Autodesk Inventor part; units mm, degrees
ref_plane "Work Plane1" through (0, 0, 0) normal (0, 0.5, 0.866) x (1, 0, 0)
ref_plane "YZ Plane" through (0, 0, 0) normal (1, 0, 0) x (0, 1, 0)
ref_plane "XZ Plane" through (0, 0, 0) normal (0, 1, 0) x (-1, 0, 0)
sketch "Sketch1" plane through (0, 0, 0) normal (0, 0, 1) x (1, 0, 0)
  line L0 (-1.7498, 0) -> (30, 0)
  line L1 (30, 0) -> (30, 7)
  line L2 (30, 7) -> (2, 7)
  line L3 (2, 7) -> (0.7731, 6.4585)
  line L4 (0.7731, 6.4585) -> (0.45, 6.4585)
  line L5 (0, 6.9085) -> (0, 10.5)
  line L6 (0, 10.5) -> (-9, 10.5)
  line L7 (-9, 10.5) -> (-9, 5.6295)
  line L8 (-9, 5.6295) -> (-5, 5.6295)
  line L9 (-5, 5.6295) -> (-1.7498, 0)
  line L10 (-16.8, 0) -> (37.8, 0)
  line L11 (0, -2.1) -> (0, 12.6)
  line L12 (2, 7) -> (0, 7) construction
  arc A0 (0, 6.9085) -> (0.45, 6.4585) centre (0.45, 6.9085) ccw
  line L13 (0, 10.5) -> (-9, 9.7126)
  point P0 (0, 6.4585)
  dimension "d1" = 28
  dimension "d2" = 1.2269
  dimension "d3" = 9
  dimension "d4" = 4
  dimension "d5" = 60
  dimension "d6" = 14
  dimension "d7" = 12.917
  dimension "d8" = 11.259
  dimension "d9" = 21
  dimension "d20" = 30
  dimension "d34" = 0.45
  dimension "d35" = 5
revolve "Body" add sketch "Sketch1" angle 360 about axis through (-1.7498, 0, 0) along (1, 0, 0)
sketch "Sketch2" plane through (-9, 0, 0) normal (-1, 0, 0) x (0, 0, 1)
  line L0 (0, -14.7) -> (0, 14.7)
  line L1 (-14.7, 0) -> (14.7, 0)
  circle A0 centre (0, 0) radius 10.5
  circle A1 centre (0, 0) radius 3.9725
  line L2 (0, 0) -> (4.8438, 8.3897) construction
  line L3 (0, 0) -> (8.7121, 5.0299) construction
  circle A2 centre (0, 0) radius 5.6295
  arc A3 (3.1732, 4.0107) -> (1.8868, 4.7534) centre (2.4303, 4.2093) ccw
  arc A4 (5.06, -0.7427) -> (5.06, 0.7427) centre (4.8605, 0) ccw
  arc A5 (3.1732, 4.0107) -> (5.06, 0.7427) centre (5.7525, 3.3212) ccw
  arc A6 (-1.8868, 4.7534) -> (-3.1732, 4.0107) centre (-2.4303, 4.2093) ccw
  arc A7 (-5.06, 0.7427) -> (-5.06, -0.7427) centre (-4.8605, 0) ccw
  arc A8 (-5.06, 0.7427) -> (-3.1732, 4.0107) centre (-5.7525, 3.3212) ccw
  arc A9 (1.8868, -4.7534) -> (3.1732, -4.0107) centre (2.4303, -4.2093) ccw
  arc A10 (5.06, -0.7427) -> (5.06, 0.7427) centre (4.8605, 0) ccw
  arc A11 (5.06, -0.7427) -> (3.1732, -4.0107) centre (5.7525, -3.3212) ccw
  arc A12 (-3.1732, -4.0107) -> (-1.8868, -4.7534) centre (-2.4303, -4.2093) ccw
  arc A13 (-3.1732, -4.0107) -> (-5.06, -0.7427) centre (-5.7525, -3.3212) ccw
  arc A14 (-5.06, 0.7427) -> (-5.06, -0.7427) centre (-4.8605, 0) ccw
  arc A15 (-1.8868, 4.7534) -> (1.8868, 4.7534) centre (0, 6.6424) ccw
  arc A16 (1.8868, -4.7534) -> (-1.8868, -4.7534) centre (0, -6.6424) ccw
  dimension "d38" = 7.945
  dimension "d39" = 30
  dimension "d40" = 60
  dimension "d42" = 0.769
extrude "Slot" add sketch "Sketch2" against normal up to next contours A2 A12 A16 L0 | L0 A16 A9 A2 | A2 A7 A13 A12 | A9 A11 A4 A2 | A2 A6 A8 A7 | A4 A5 A3 A2 | A2 L0 A15 A6 | A2 A3 A15 L0
revolve "Taper" cut sketch "Sketch1" angle 360 about axis through (0, 0, 0) along (1, 0, 0) contours L13 L7 L6
fillet "Fillet1" radius 0.9 1 edges at (-9, -9.7126, 0)
thread "Thread"
chamfer "Chamfer1" distance 1.2269 distance2 1.227 1 edges at (30, -7, 0) measured on face at (30, -0.3293, 1.9203)
ref_plane "Work Plane1" through (0, 0, 0) normal (0, 0.5, 0.866) x (1, 0, 0)
equation "\"d1\" = GEL"
equation "\"d2\" = GAL"
equation "\"d3\" = KOH"
equation "\"d4\" = INTI"
equation "\"d6\" = GD"
equation "\"d7\" = BDM"
equation "\"d8\" = E0"
equation "\"d9\" = KOD"
equation "\"d20\" = NLG"
equation "\"d34\" = R"
equation "\"d38\" = SW"
equation "\"d42\" = RRK"
equation "\"d17\" = RR"
equation "\"d13\" = GEL"
equation "\"d15\" = -0.5 * SPD + 0.5 * GD"
equation "\"GD\" = NND"
equation "\"NLG\" = 30"
equation "\"GEL\" = 28"
equation "\"KOD\" = 21"
equation "\"KOH\" = 9"
equation "\"INTI\" = 4"
equation "\"GAL\" = 0.61345 * PTC"
equation "\"GUL\" = 0.61345 * PTC"
equation "\"BDM\" = 12.917"
equation "\"SW\" = 7.945"
equation "\"RR\" = 0.9"
equation "\"SPD\" = NND - 1.2269 * PTC"
equation "\"R\" = 0.45"
equation "\"E0\" = 11.259"
equation "\"RRK\" = 0.769"
equation "\"PHH\" = 0"
equation "\"GD1\" = THREADDIA - 1.2269 * PTC"
equation "\"THREADDIA\" = 14"
equation "\"FAWI\" = 90deg"
equation "\"ANG\" = 120deg"
equation "\"PTC\" = 2"
equation "\"NND\" = 14"
equation "\"TOA\" = 30deg"
equation "\"KEWI\" = 5deg"
properties part number "Screw GB/T 2171.1 M14 x 30" material "Steel, Mild"
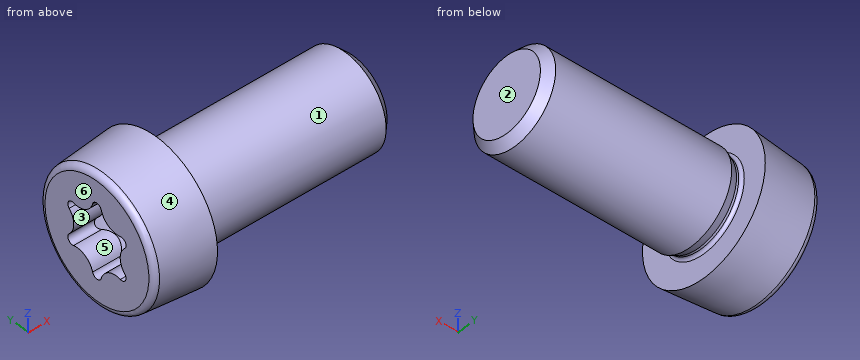
Build history of the part. All positions in model axes, mm. Face numbers are marked on the shaded views. A direction names the side the tool comes from. Coordinates: 2 decimals unless noted, no trailing zeros. Write each loop counter-clockwise with the first axis right and the second up, starting at its lowest first coordinate (ties: lowest second). Pieces come first, ordered by that corner, then holes.
(1) Mould opens along Z. For the marked faces 3, 4, 5 and 6 say: pulls with the +Z half, pulls with the -Z half, needs draft (parallel to the pull), parting line crosses it, or undercut.
(2) Drill centre lines: line 1 (Z direction, x = 20.5, y = 0); line 2 (X direction, y = -5.25, z = 7); line 3 (Y direction, x = -4.5, z = 4). Where is each one in solid material? Low to high.
(3) Pin check, flat tips, straight feed: pin 1 Ø1.5 at (x, z) = (25, -7) entering from -Y; pin 2 Ø3 at (x, z) = (15, 2.5) entering from +Y; pin 3 Ø5 at (x, z) = (25.5, 8) entering from -Y. Stop position of each tip, or through.
(4) 3-axis set-ups, long thin cutter, end or side, ignore diameter. For the marked faces 1 and 2: which of +Z, -Z, +X, -X, +Y, -Y reach the whole face in a straight line?
(5) Cut at B-B on x = 8. List the corners of the cut face in (y, z).
(6) Cut at A-A on x = -3.5. List the corners of the cut face in (y, z).
Working result:
1. face 3: undercut
1. face 4: parting line crosses it
1. face 5: undercut
1. face 6: needs draft
2. line 1: z = -7 to 7
2. line 2: x = -9 to 0
2. line 3: y = -9.28 to -1.31, 1.31 to 9.28
3. pin 1: stops at y = -3.15
3. pin 2: stops at y = 6.93
3. pin 3: stops at y = -4.33
4. face 1: +X
4. face 2: +Z, -Z, +X, +Y, -Y
5. outline: circle Ø14 at (0, 0)
6. outline: circle Ø20.39 at (0, 0); hole circle Ø6.06 at (0, 0)
